Geometry: see drawing. Coordinates: mm, zero at the bounding-box minimum. Give positions to 0.01 mm unless a question says otherwise; leave off trailing zeros. Write each loop counter-clockwise with the first axis right and the second up, starting at its lowest first coordinate (ties: lowest second). Pieces come first, ordered by that corner, then holes. Notation, with made-up numbers: (87, 21) -> (143, 21) arc R19 cw to (143, 51) -> close; hole circle Ø9 at (11.25, -10.75). An arc over 180 degrees is marked (long way). Use one line per item in the form item = value. Start each with the question number.
(1) First-contact query: P1, Ø6.5, axis at x = 12.7, z = 88.9, coming from the +Y side. Flat tip, straight axial feed; report the tip coordinate or a pass-through.
(2) Cut plane B-B, the plane x = 12.5. Output: boundary loops of the cut face in (y, z), and give its area (3 significant figures).
(3) Material intervals for line 1 along X through (y, z) = (3, 88.9); line 2 along Z through (x, y) = (12.7, 3.25), sorted ascending. Write a range as from..to.
(4) Cut plane A-A, the plane z = 88.9. Output: boundary loops of the cut face in (x, y).
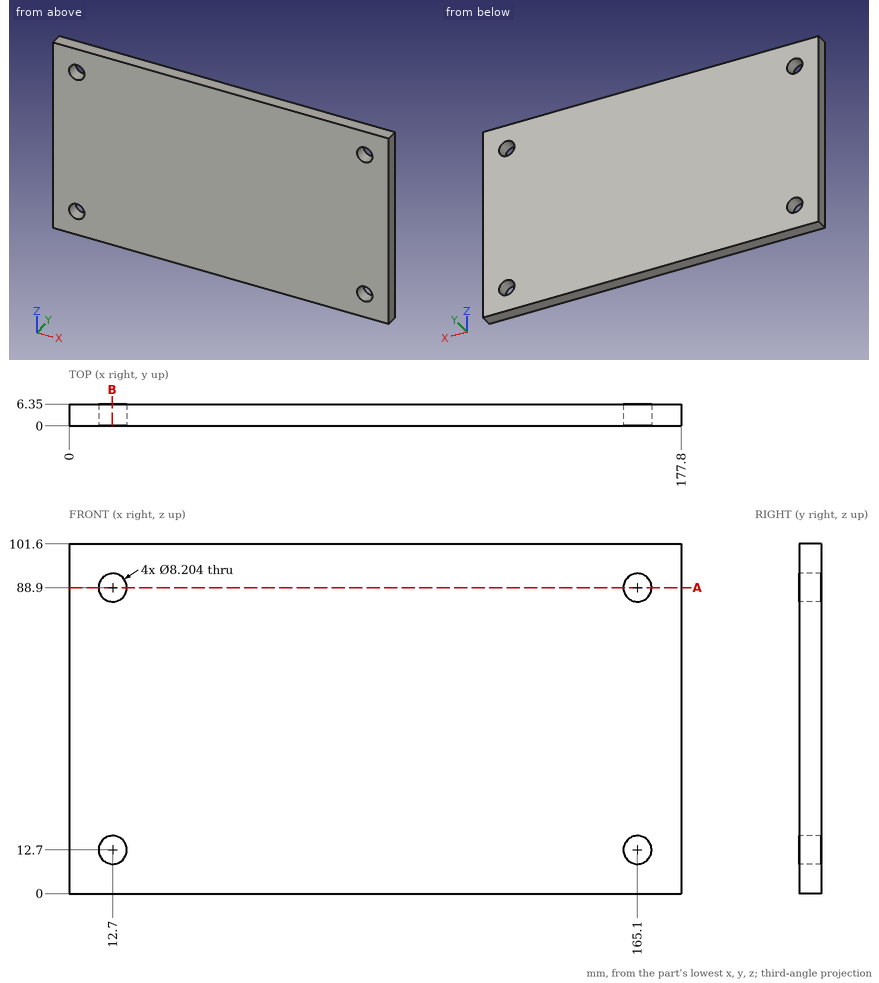
Geometry says:
q1.P1 = through
q2.outline = (0, 0) -> (6.35, 0) -> (6.35, 8.6) -> (0, 8.6) -> close; (0, 16.8) -> (6.35, 16.8) -> (6.35, 84.8) -> (0, 84.8) -> close; (0, 93) -> (6.35, 93) -> (6.35, 101.6) -> (0, 101.6) -> close
q2.area = 541 mm^2
q3.line_1 = 0..8.6, 16.8..161, 169.2..177.8
q3.line_2 = 0..8.6, 16.8..84.8, 93..101.6
q4.outline = (0, 0) -> (8.6, 0) -> (8.6, 6.35) -> (0, 6.35) -> close; (16.8, 0) -> (161, 0) -> (161, 6.35) -> (16.8, 6.35) -> close; (169.2, 0) -> (177.8, 0) -> (177.8, 6.35) -> (169.2, 6.35) -> close
